```python
from build123d import *

# Parameters (mm, degrees)
F0_W      = 5.5
F0_H      = 4.2
F1_DEPTH  = 7
F2_W      = 0.8
F2_H      = 0.95
F3_DEPTH  = 5
F1_FACE_W = 5.5
F1_FACE_H = 4.2
F4_DEPTH  = 1
F4_TAPER  = -45
F6_R      = 0.5


# Not quite as in the source:
# - a feature of the source that left no trace in its solid (it failed there, or was rolled back) is left out


with BuildPart() as f1:
    # F0 (on Top) → F1 (new body)
    with BuildSketch(Plane.XY):
        Rectangle(F0_W, F0_H)
    extrude(amount=F1_DEPTH)

    # F2 (on Top) → F3 (cut)
    with BuildSketch(Plane.XY):
        with Locations((-1.2, 0)):
            Rectangle(F2_W, F2_H)
    extrude(amount=F3_DEPTH, mode=Mode.SUBTRACT)

    # F1_face (on face) → F4 (join)
    with BuildSketch(Plane.XY.offset(7)):
        Rectangle(F1_FACE_W, F1_FACE_H)
    extrude(amount=F4_DEPTH, taper=F4_TAPER)

    # F6
    f6_edges = [f1.edges().sort_by_distance(p)[0] for p in [
        (0, -3.1, 8),
        (3.75, 0, 8),
        (0, 3.1, 8),
        (-3.75, 0, 8),
    ]]
    fillet(f6_edges, radius=F6_R)


solid = f1.part
```
Can you work these out from the model? Positions are in its coordinate system, mm. A direction names the side the tool comes from. Give positions to 0.01 mm unless a question says otherwise; leave off trailing zeros. Order: outer loops, then holes, each group sorted by start corner. A loop starts at its lowest first (then second) coordinate and runs counter-clockwise, first axis right, second up. Notation, with made-up numbers: M 64.25,-6 L 84.25,-6 A34 cw 84.25,25 Z; hole C 38.5,66.25 d11. An arc over 180 degrees is marked long. One line per item, written item: value.
1) I want a section at A-A, the plane z = 2. List the corners of the cut face in (x, y) for me (3 decimals), plus the area to 3 significant figures.
Answer sheet:
outline: M -2.75,-2.1 L 2.75,-2.1 L 2.75,2.1 L -2.75,2.1 Z; hole M -1.6,-0.475 L -0.8,-0.475 L -0.8,0.475 L -1.6,0.475 Z
area: 22.3 mm^2
2) I want a section at B-B, the plane z = 5.25. List the corners of the cut face in (x, y) for me.
Answer sheet:
outline: M -2.75,-2.1 L 2.75,-2.1 L 2.75,2.1 L -2.75,2.1 Z
3) We'd pull the mould along X, two halves only. Please class faces 1 (the face through (2.75, 0, 3)), 2 (the face through (-0.8, 0, 2)), 3 (the face through (0, 2.1, 3)): released by +X, released by -X, zero draft, split by the parting line, or undercut.
Answer sheet:
face 1: released by +X
face 2: undercut
face 3: zero draft
4) For P1, Ø1.3, axis at y = -1, z = 2.5, coming from the -X side; P2, Ø3, axis at x = 2, z = 1, coming from the -Y side; P3, Ø2, axis at y = 1.5, z = 5, coming from the +X side; P4, Ø2, axis at x = 2, y = 2, coming from the -Z side, each with a flat end and sliding along its axis, tell me the tip position at first contact or that it passes through.
Answer sheet:
P1: stops at x = -2.75
P2: stops at y = -2.1
P3: stops at x = 2.75
P4: stops at z = 0
5) On a 3-axis mill with a long thin cutter (end or side, diameter ignored), from which of +Z, -Z, +X, -X, +Y, -Y can I reach the whole of each face in a straight line? I mean faces 4 (the face through (0, 0, 0)), 5 (the face through (-1.6, 0, 2)), 6 (the face through (-2.75, 0, 3)), 7 (the face through (0, 0, 8)), 8 (the face through (0, -2.1, 3)). Say none if no direction works.
Answer sheet:
face 4: -Z, +X, -X, +Y, -Y
face 5: -Z
face 6: -Z, -X, +Y, -Y
face 7: +Z, +X, -X, +Y, -Y
face 8: -Z, +X, -X, -Y
6) Please list where these lines run through material, in increasing order: line 1 along Y through (x, z) = (-1.25, 2.25) (3 decimals); line 2 along X through (y, z) = (-0.75, 0.5); line 3 along Y through (x, z) = (2.25, 6.75).
Answer sheet:
line 1: y = -2.1 to -0.475, 0.475 to 2.1
line 2: x = -2.75 to 2.75
line 3: y = -2.1 to 2.1
